```python
from build123d import *
from build123d.topology import SkipClean

# Parameters (mm, degrees)
SKETCH2_R           = 1
SKETCH2_R_2         = 26
BOSS_EXTRUDE1_DEPTH = 10
SKETCH3_R           = 31
SKETCH3_R_2         = 5.1
BOSS_EXTRUDE2_DEPTH = 2
BOSS_EXTRUDE3_DEPTH = 6.5
SKETCH5_R           = 12.5
SKETCH5_R_2         = 5.1
BOSS_EXTRUDE4_DEPTH = 2
FILLET1_R           = 1
BOSS_EXTRUDE5_START = 6.5
BOSS_EXTRUDE5_DEPTH = 6.5
FILLET2_R           = 1
CUT_EXTRUDE1_START  = -9
SKETCH7_R           = 4
CUT_EXTRUDE1_DEPTH  = 9
BOSS_EXTRUDE6_START = 10
BOSS_EXTRUDE6_DEPTH = 10
CIRPATTERN1_COUNT   = 4
SKETCH12_R          = 26
CUT_EXTRUDE2_DEPTH  = 3


with BuildPart() as part:
    # Sketch2 → Boss-Extrude1 (new body)
    with BuildSketch(Plane(origin=(0, 0, 0), x_dir=(1, 0, 0), z_dir=(0, 1, 0))):
        with BuildLine():
            ThreePointArc((3.991666658, 30.741935484), (0, 35), (-3.991666658, 30.741935484))
            ThreePointArc((-3.991666658, 30.741935484), (-21.920310217, 21.920310217), (-30.741935484, 3.991666658))
            ThreePointArc((-30.741935484, 3.991666658), (-35, 0), (-30.741935484, -3.991666658))
            ThreePointArc((-30.741935484, -3.991666658), (-21.920310217, -21.920310217), (-3.991666658, -30.741935484))
            ThreePointArc((-3.991666658, -30.741935484), (0, -35), (3.991666658, -30.741935484))
            ThreePointArc((3.991666658, -30.741935484), (21.920310217, -21.920310217), (30.741935484, -3.991666658))
            ThreePointArc((30.741935484, -3.991666658), (35, 0), (30.741935484, 3.991666658))
            ThreePointArc((30.741935484, 3.991666658), (21.920310217, 21.920310217), (3.991666658, 30.741935484))
        make_face()
        with Locations(Location((0, 31, 0), (0, 0, 270))):
            Circle(SKETCH2_R, mode=Mode.SUBTRACT)
        with Locations(Location((31, 0, 0), (0, 0, 270))):
            Circle(SKETCH2_R, mode=Mode.SUBTRACT)
        with Locations(Location((0, -31, 0), (0, 0, 270))):
            Circle(SKETCH2_R, mode=Mode.SUBTRACT)
        with Locations(Location((-31, 0, 0), (0, 0, 270))):
            Circle(SKETCH2_R, mode=Mode.SUBTRACT)
        with Locations(Location((0, 0, 0), (0, 0, 270))):
            Circle(SKETCH2_R_2, mode=Mode.SUBTRACT)
    extrude(amount=BOSS_EXTRUDE1_DEPTH)

    # Sketch3 → Boss-Extrude2 (add)
    with BuildSketch(Plane(origin=(0, 10, 0), x_dir=(1, 0, 0), z_dir=(0, 1, 0))):
        with Locations(Location((0, 0, 0), (0, 0, 88.151668903))):
            Circle(SKETCH3_R)
        with Locations(Location((0, 0, 0), (0, 0, 270))):
            Circle(SKETCH3_R_2, mode=Mode.SUBTRACT)
    extrude(amount=BOSS_EXTRUDE2_DEPTH)

    # Sketch4 → Boss-Extrude3 (add)
    with BuildSketch(Plane(origin=(0, 12, 0), x_dir=(1, 0, 0), z_dir=(0, 1, 0))):
        Polygon((-5.022947342, 8.7), (-10.045894684, 0), (-5.022947342, -8.7), (5.022947342, -8.7), (5.022947342, -10.7), (-6.17764788, -10.7), (-12.355295761, 0), (-6.17764788, 10.7), (5.022947342, 10.7), (5.022947342, 8.7), align=None)
    extrude(amount=BOSS_EXTRUDE3_DEPTH)

    # Sketch5 → Boss-Extrude4 (add)
    with BuildSketch(Plane(origin=(0, 18.5, 0), x_dir=(1, 0, 0), z_dir=(0, 1, 0))):
        with Locations(Location((0, 0, 0), (0, 0, 270))):
            Circle(SKETCH5_R)
        with Locations(Location((0, 0, 0), (0, 0, 270))):
            Circle(SKETCH5_R_2, mode=Mode.SUBTRACT)
    extrude(amount=BOSS_EXTRUDE4_DEPTH)

    # Fillet1
    fillet1_edges = [part.edges().sort_by_distance(p)[0] for p in [
        (0, 12, -8.7),
        (0, 12, 8.7),
        (-7.534421013, 12, 4.35),
        (-7.534421013, 12, -4.35),
        (-10.045894684, 15.25, 0),
        (0, 18.5, -8.7),
        (0, 18.5, 8.7),
        (-7.534421013, 18.5, 4.35),
        (-7.534421013, 18.5, -4.35),
    ]]
    fillet(fillet1_edges, radius=FILLET1_R)

    # Sketch6 → Boss-Extrude5 (add)
    with SkipClean():  # the faces are left unmerged after this step: merging them gives an invalid solid
        with BuildSketch(Plane.XZ.offset(-18.5).offset(BOSS_EXTRUDE5_START)):
            with BuildLine():
                Line((-6.17764788, -10.7), (-12.355295761, 0))
                Line((-12.355295761, 0), (-6.17764788, 10.7))
                Line((-6.17764788, 10.7), (5.022947342, 10.7))
                Line((5.022947342, 10.7), (5.022947342, 11.446396813))
                ThreePointArc((5.022947342, 11.446396813), (-12.5, 0), (5.022947342, -11.446396813))
                Line((5.022947342, -11.446396813), (5.022947342, -10.7))
                Line((5.022947342, -10.7), (-6.17764788, -10.7))
            make_face()
        extrude(amount=-BOSS_EXTRUDE5_DEPTH)

    # Fillet2
    fillet2_edges = [part.edges().sort_by_distance(p)[0] for p in [
        (-12.5, 12, 0),
        (5.022947342, 12, -9.2),
        (5.022947342, 12, 9.2),
    ]]
    fillet(fillet2_edges, radius=FILLET2_R)

    # Sketch7 → Cut-Extrude1 (cut)
    with BuildSketch(Plane(origin=(0, 12, 0), x_dir=(1, 0, 0), z_dir=(0, 1, 0)).offset(CUT_EXTRUDE1_START)):
        with Locations((0, -31)):
            Circle(SKETCH7_R)
        with Locations((31, 0)):
            Circle(SKETCH7_R)
        with Locations((0, 31)):
            Circle(SKETCH7_R)
        with Locations((-31, 0)):
            Circle(SKETCH7_R)
    extrude(amount=CUT_EXTRUDE1_DEPTH, mode=Mode.SUBTRACT)

    # Sketch10 → Boss-Extrude6 (add)
    with BuildSketch(Plane.XZ.offset(-10).offset(BOSS_EXTRUDE6_START)):
        with BuildLine():
            Line((-4, 25.690465157), (-4, 15))
            Line((-4, 15), (4, 15))
            Line((4, 15), (4, 25.690465157))
            ThreePointArc((4, 25.690465157), (0, 26), (-4, 25.690465157))
        make_face()
    boss_extrude6 = extrude(amount=-BOSS_EXTRUDE6_DEPTH)

    # CirPattern1: Boss-Extrude6 ×4 about axis
    cirpattern1_axis = Axis((0, 0, 0), (0, 1, 0))
    for i in range(1, CIRPATTERN1_COUNT):
        add(boss_extrude6.rotate(cirpattern1_axis, i * 360 / CIRPATTERN1_COUNT))

    # Sketch12 → Cut-Extrude2 (cut)
    with SkipClean():  # the faces are left unmerged after this step: merging them gives an invalid solid
        with BuildSketch(Plane.XZ):
            with Locations(Location((0, 0, 0), (0, 0, 261.150116902))):
                Circle(SKETCH12_R)
        extrude(amount=-CUT_EXTRUDE2_DEPTH, mode=Mode.SUBTRACT)
    add(part.part.scale(1), mode=Mode.REPLACE)  # the faces are merged on a copy


solid = part.part
```
For this review, take the finished solid that the model builds, in its own axes (mm). A direction names the side the tool comes from. Round coordinates to 2 decimals unless told otherwise and drop trailing zeros. Write each loop counter-clockwise with the first axis right and the second up, starting at its lowest first coordinate (ties: lowest second). Pieces come first, ordered by that corner, then holes. Notation, with made-up numbers: M -9.5,2 L 37.5,2 A11 cw 37.5,12 Z; hole C 22,42.25 d1. An arc over 180 degrees is marked long. One line per item, written item: value. Start each with the question number.
(1) We need section A-A (y = 9). Give the boundary of the cut face in (x, z).
(2) Wall thickness on line 1 (X direction, y = 1.1, z = 0); line 2 (X direction, y = 6.25, z = 21): over which ranges is each line inside the solid? List them lowest first.
(3) The part is to be moulded in two halves that separate along Z. For faces 1 (the flat face through (5.023, 16, -10)), 2 (the cylindrical face through (1.532, 19.486, 4.864)), say which applies: released by +Z, released by -Z, zero draft, split by the parting line, or undercut.
(4) We need section D-D (x = 17.5). Give the boundary of the cut face in (y, z).
(5) We need section C-C (x = 0). Count the separate pieces of the cut face and the enclosed holes in it, and give its area (3 significant figures).
(6) We need section B-B (y = 14.5). Give the boundary of the cut face in (x, z), and give its area (3 significant figures).
(7) Machinability: for faces 3 (the flat face through (-20, 6, 4)), 4 (the cylindrical face through (-30, 1, 0)), 5 (the cylindrical face through (-7.163, 18.215, -4.392)), which of the approach directions +Z, -Z, +X, -X, +Y, -Y give a long, thin tool a straight path to every point of the face, cutting with its end or side? Answer none if there is none.
(8) Insertion check: pin 1 (7.5 mm diameter, centred on x = 19, y = 7, fed in from -Z); pin 2 (8 mm diameter, centred on x = 0, z = 0, fed in from -Y); pin 3 (6 mm diameter, centred on y = 13.5, z = 20.5, fed in from +X); pin 4 (2 mm diameter, centred on y = 6.5, z = 19, fed in from +X). Each pin has a flat end and moves straight along its axis. Give the tip position at first contact, or say it passes through.
Result:
1. outline: M -30.74,-3.99 A31 ccw -3.99,-30.74 A4 cw 3.99,-30.74 A31 ccw 30.74,-3.99 A4 cw 30.74,3.99 A31 ccw 3.99,30.74 A4 cw -3.99,30.74 A31 ccw -30.74,3.99 A4 cw Z; hole M -25.69,-4 A26 ccw -4,-25.69 L -4,-15 L 4,-15 L 4,-25.69 A26 ccw 25.69,-4 L 15,-4 L 15,4 L 25.69,4 A26 ccw 4,25.69 L 4,15 L -4,15 L -4,25.69 A26 ccw -25.69,4 L -15,4 L -15,-4 Z
2. line 1: -35 to -32, -30 to -26, 26 to 30, 32 to 35
2. line 2: -22.8 to -15.33, -4 to 4, 15.33 to 22.8
3. face 1: zero draft
3. face 2: undercut
4. outline: M 0,-25.59 L 12,-25.59 L 12,25.59 L 0,25.59 L 0,19.23 L 10,19.23 L 10,4 L 3,4 L 3,-4 L 10,-4 L 10,-19.23 L 0,-19.23 Z
5. separate pieces: 4
5. enclosed holes: 0
5. area: 378 mm²
6. outline: M -9.76,-0.5 A1 cw -9.76,0.5 L -5.02,8.7 L 5.02,8.7 L 5.02,11.45 A12.5 ccw long 5.02,-11.45 L 5.02,-8.7 L -5.02,-8.7 Z
6. area: 149 mm²
7. face 3: -Y
7. face 4: +Y, -Y
7. face 5: +X
8. pin 1: z = -26.99
8. pin 2: through
8. pin 3: x = 25.31
8. pin 4: x = 25.24
